```python
from build123d import *

# Parameters (mm, degrees)
SKETCH_R      = 3.05
SKETCH_R_2    = 1.85
SKETCH_W      = 30.3
SKETCH_H      = 15.35
SKETCH_W_2    = 25
SKETCH_H_2    = 3
SKETCH_W_3    = 3
SKETCH_H_3    = 25
EXTRUDE_DEPTH = 3


with BuildPart() as part:
    # Sketch → Extrude (new body)
    with BuildSketch(Plane.XY):
        with BuildLine():
            ThreePointArc((0, 106), (-4.242641, 104.242641), (-6, 100))
            Line((-6, 100), (-6, 0))
            ThreePointArc((-6, 0), (-4.242641, -4.242641), (0, -6))
            Line((0, -6), (100, -6))
            ThreePointArc((100, -6), (104.242641, -4.242641), (106, 0))
            Line((106, 0), (106, 100))
            ThreePointArc((106, 100), (104.242641, 104.242641), (100, 106))
            Line((0, 106), (100, 106))
        make_face()
        with Locations((17.7, 10.3)):
            Circle(SKETCH_R, mode=Mode.SUBTRACT)
        with Locations((35.2, 10.3)):
            Circle(SKETCH_R, mode=Mode.SUBTRACT)
        with Locations((52.7, 10.3)):
            Circle(SKETCH_R, mode=Mode.SUBTRACT)
        with Locations((76.6, 10.3)):
            Circle(SKETCH_R, mode=Mode.SUBTRACT)
        with Locations((63.4, 36.45)):
            Circle(SKETCH_R, mode=Mode.SUBTRACT)
        with Locations((4, 96)):
            Circle(SKETCH_R_2, mode=Mode.SUBTRACT)
        with Locations((96, 96)):
            Circle(SKETCH_R_2, mode=Mode.SUBTRACT)
        with Locations((96, 4)):
            Circle(SKETCH_R_2, mode=Mode.SUBTRACT)
        with Locations((4, 4)):
            Circle(SKETCH_R_2, mode=Mode.SUBTRACT)
        with Locations((35.195, 35.755)):
            Rectangle(SKETCH_W, SKETCH_H, mode=Mode.SUBTRACT)
        with Locations((27.5, 101.5)):
            Rectangle(SKETCH_W_2, SKETCH_H_2, mode=Mode.SUBTRACT)
        with Locations((72.5, 101.5)):
            Rectangle(SKETCH_W_2, SKETCH_H_2, mode=Mode.SUBTRACT)
        with Locations((101.5, 72.5)):
            Rectangle(SKETCH_W_3, SKETCH_H_3, mode=Mode.SUBTRACT)
        with Locations((101.5, 27.5)):
            Rectangle(SKETCH_W_3, SKETCH_H_3, mode=Mode.SUBTRACT)
        with Locations((72.5, -1.5)):
            Rectangle(SKETCH_W_2, SKETCH_H_2, mode=Mode.SUBTRACT)
        with Locations((27.5, -1.5)):
            Rectangle(SKETCH_W_2, SKETCH_H_2, mode=Mode.SUBTRACT)
        with Locations((-1.5, 27.5)):
            Rectangle(SKETCH_W_3, SKETCH_H_3, mode=Mode.SUBTRACT)
        with Locations((-1.5, 72.5)):
            Rectangle(SKETCH_W_3, SKETCH_H_3, mode=Mode.SUBTRACT)
    extrude(amount=EXTRUDE_DEPTH)


solid = part.part
```
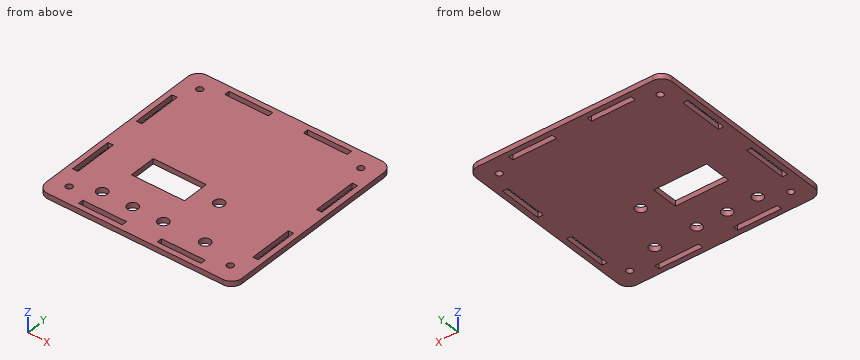
Model file for the job. Use its own axes, mm. Coordinates: 2 decimals unless noted, no trailing zeros. Loops run counter-clockwise (first coordinate to the right, second up) from the corner with the lowest first, then second, coordinate; pieces in that order, holes last. Notation, with made-up numbers: M -6.75,33.5 L 11.25,33.5 A19 ccw 11.25,54.5 Z; hole C 19.25,62 d7. An arc over 180 degrees is marked long. Use CSV: the item, a comma, the result in double quotes. Start each with the question number.
1. Band-saw the part on D-D, the plane y = 10.3. List the corners of the cut face in (x, z), then the cut area to 3 significant figures.
2. Band-saw the part on A-A, the plane x = 96. List the corners of the cut face in (y, z), then the cut area to 3 significant figures.
3. Band-saw the part on B-B, the plane y = 74.5. List the corners of the cut face in (x, z), then the cut area to 3 significant figures.
4. Probe probe 1 along X at (y, z) = (23, 1.65); probe 2 along Y at (x, z) = (4, 1.5); probe 3 along Y at (x, z) = (17.7, 0.6). List the from-to ranges inside material, lowest first. Write a range as [from, to].
5. Band-saw the part on C-C, the plane x = 63.4. List the corners of the cut face in (y, z), then the cut area to 3 significant figures.
6. Flat gauge pins, fed straight in: pin 1 (1.5 mm diameter, centred on x = -1.5, z = 1, fed in from -Y); pin 2 (0.9 mm diameter, centred on y = -2, z = 1.5, fed in from +X); pin 3 (0.9 mm diameter, centred on y = -1.5, z = 1, fed in from -X); pin 4 (3.5 mm diameter, centred on x = 52.7, y = 10.3, fed in from -Z). Where does each tip first touch, or does it go through?
Entries:
1,outline,"M -6,0 L 14.65,0 L 14.65,3 L -6,3 Z; M 20.75,0 L 32.15,0 L 32.15,3 L 20.75,3 Z; M 38.25,0 L 49.65,0 L 49.65,3 L 38.25,3 Z; M 55.75,0 L 73.55,0 L 73.55,3 L 55.75,3 Z; M 79.65,0 L 106,0 L 106,3 L 79.65,3 Z"
1,area,"263 mm2"
2,outline,"M -6,0 L 2.15,0 L 2.15,3 L -6,3 Z; M 5.85,0 L 94.15,0 L 94.15,3 L 5.85,3 Z; M 97.85,0 L 106,0 L 106,3 L 97.85,3 Z"
2,area,"314 mm2"
3,outline,"M -6,0 L -3,0 L -3,3 L -6,3 Z; M 0,0 L 100,0 L 100,3 L 0,3 Z; M 103,0 L 106,0 L 106,3 L 103,3 Z"
3,area,"318 mm2"
4,probe 1,"x = [-6, -3], [0, 100], [103, 106]"
4,probe 2,"y = [-6, 2.15], [5.85, 94.15], [97.85, 106]"
4,probe 3,"y = [-6, -3], [0, 7.25], [13.35, 100], [103, 106]"
5,outline,"M -6,0 L -3,0 L -3,3 L -6,3 Z; M 0,0 L 33.4,0 L 33.4,3 L 0,3 Z; M 39.5,0 L 100,0 L 100,3 L 39.5,3 Z; M 103,0 L 106,0 L 106,3 L 103,3 Z"
5,area,"300 mm2"
6,pin 1,"stops at y = -5.95"
6,pin 2,"stops at x = 105.8"
6,pin 3,"stops at x = -5.91"
6,pin 4,"passes through"
